Could you check a few things on this model? Use its own coordinates, in mm. A direction names the side the tool comes from. Give positions to 0.01 mm unless a question says otherwise; leave off trailing zeros. Write each loop counter-clockwise with the first axis right and the second up, starting at its lowest first coordinate (ties: lowest second). Pieces come first, ordered by that corner, then holes. Notation, with made-up numbers: (10.5, 69) - (54.5, 69) arc R33 ccw to (54.5, 97) - close; hole circle Ø6 at (-24, -25.75). An arc over 180 degrees is marked (long way). Write item = value, one per line.
from build123d import *

# Parameters (mm, degrees)
F0_W     = 85
F0_H     = 41
F0_R     = 1.8
F0_W_2   = 73
F0_H_2   = 25.4
F1_DEPTH = 3.3
F0_W_3   = 65
F0_H_3   = 15
F2_DEPTH = 5
F3_R     = 5
F4_SIZE  = 3
F5_SIZE  = 1
F6_SIZE  = 1.5


with BuildPart() as f1:
    # F0 (on Top) → F1 (new body)
    with BuildSketch(Plane.XY):
        Rectangle(F0_W, F0_H)
        with Locations((-37.5, -15.5)):
            Circle(F0_R, mode=Mode.SUBTRACT)
        with Locations((37.5, -15.5)):
            Circle(F0_R, mode=Mode.SUBTRACT)
        with Locations((-37.5, 15.5)):
            Circle(F0_R, mode=Mode.SUBTRACT)
        Rectangle(F0_W_2, F0_H_2, mode=Mode.SUBTRACT)
        with Locations((37.5, 15.5)):
            Circle(F0_R, mode=Mode.SUBTRACT)
    extrude(amount=F1_DEPTH)

    # F0 (on Top) → F2 (join)
    with BuildSketch(Plane.XY):
        Rectangle(F0_W, F0_H)
        with Locations((-37.5, -15.5)):
            Circle(F0_R, mode=Mode.SUBTRACT)
        with Locations((37.5, -15.5)):
            Circle(F0_R, mode=Mode.SUBTRACT)
        with Locations((-37.5, 15.5)):
            Circle(F0_R, mode=Mode.SUBTRACT)
        Rectangle(F0_W_2, F0_H_2, mode=Mode.SUBTRACT)
        with Locations((37.5, 15.5)):
            Circle(F0_R, mode=Mode.SUBTRACT)
        Rectangle(F0_W_2, F0_H_2)
        with Locations((0, -1)):
            Rectangle(F0_W_3, F0_H_3, mode=Mode.SUBTRACT)
    extrude(amount=-F2_DEPTH)

    # F3
    f3_edges = [f1.edges().sort_by_distance(p)[0] for p in [
        (-42.5, 20.5, -0.85),
        (-42.5, -20.5, -0.85),
        (42.5, 20.5, -0.85),
        (42.5, -20.5, -0.85),
    ]]
    fillet(f3_edges, radius=F3_R)

    # F4
    f4_edges = [f1.edges().sort_by_distance(p)[0] for p in [
        (0, -8.5, -5),
        (-32.5, -1, -5),
        (0, 6.5, -5),
        (32.5, -1, -5),
    ]]
    chamfer(f4_edges, length=F4_SIZE)

    # F5
    f5_edges = [f1.edges().sort_by_distance(p)[0] for p in [
        (-42.5, 0, -5),
    ]]
    chamfer(f5_edges, length=F5_SIZE)

    # F6
    f6_edges = [f1.edges().sort_by_distance(p)[0] for p in [
        (-39.3, 15.5, -5),
        (-39.3, -15.5, -5),
        (35.7, -15.5, -5),
        (35.7, 15.5, -5),
    ]]
    chamfer(f6_edges, length=F6_SIZE)


solid = f1.part
1. If we section it at C-C, the plane y = 3: Please give me the cut outline in (x, z), and give its area (3 significant figures).
Filled sheet:
outline = (-42.5, -4) - (-41.5, -5) - (-35.5, -5) - (-32.5, -2) - (-32.5, 0) - (-36.5, 0) - (-36.5, 3.3) - (-42.5, 3.3) - close; (32.5, -2) - (35.5, -5) - (41.5, -5) - (42.5, -4) - (42.5, 3.3) - (36.5, 3.3) - (36.5, 0) - (32.5, 0) - close
area = 130 mm2
2. If we section it at A-A, the plane z = 1: Please give me the cut outline in (x, y), and give its area (3 significant figures).
Filled sheet:
outline = (-42.5, -15.5) arc R5 ccw to (-37.5, -20.5) - (37.5, -20.5) arc R5 ccw to (42.5, -15.5) - (42.5, 15.5) arc R5 ccw to (37.5, 20.5) - (-37.5, 20.5) arc R5 ccw to (-42.5, 15.5) - close; hole circle Ø3.6 at (-37.5, -15.5); hole circle Ø3.6 at (-37.5, 15.5); hole (-36.5, -12.7) - (36.5, -12.7) - (36.5, 12.7) - (-36.5, 12.7) - close; hole circle Ø3.6 at (37.5, -15.5); hole circle Ø3.6 at (37.5, 15.5)
area = 1,570 mm2
3. Thinking about a two-plate mould opening in Y: for faces 1 (the face through (-1, -20.5, 0)), 2 (the face through (41.07, 19, -0.4)), 3 (the face through (-1, -13, 3.3)), 4 (the face through (0, 6.5, -1)), which applies, pulls with the +Y half, pulls with the -Y half, needs draft (parallel to the pull), parting line crosses it, or undercut?
Filled sheet:
face_1 = pulls with the -Y half
face_2 = pulls with the +Y half
face_3 = needs draft
face_4 = undercut
4. If we section it at B-B, the plane x = -14: Please give me the cut outline in (y, z), and give its area (3 significant figures).
Filled sheet:
outline = (-20.5, -4) - (-19.5, -5) - (-11.5, -5) - (-8.5, -2) - (-8.5, 0) - (-12.7, 0) - (-12.7, 3.3) - (-20.5, 3.3) - close; (6.5, -2) - (9.5, -5) - (19.5, -5) - (20.5, -4) - (20.5, 3.3) - (12.7, 3.3) - (12.7, 0) - (6.5, 0) - close
area = 171 mm2
5. I need wall thicknesses on line 1 (Y direction, x = 37.5, z = -2.65); line 2 (X direction, y = -3.5, z = -1.25); line 3 (Y direction, x = -14, z = 1.5). Which ranges of each line are inside material? Lowest first, please.
Filled sheet:
line_1 = -20.5 to -17.3, -13.7 to 13.7, 17.3 to 20.5
line_2 = -42.5 to -32.5, 32.5 to 42.5
line_3 = -20.5 to -12.7, 12.7 to 20.5
6. Which directions (+Z, -Z, +X, -X, +Y, -Y) give clear straight access to the entire face, cutting with the end or side of a thin tool? Please do faces 5 (the face through (0, -8.5, -1)), 6 (the face through (42.5, 0, 0)), 7 (the face through (-36.5, 0, 2)), 8 (the face through (-0.5, -10, -3.5)), 9 (the face through (41.07, -19, -0.3)).
Filled sheet:
face_5 = +Z, -Z
face_6 = +Z, -Z, +X, +Y, -Y
face_7 = +Z
face_8 = -Z
face_9 = +Z, -Z, +X, -Y
7. For pin 1 (4.5 mm diameter, centred on x = 37.5, y = -15.5, fed in from +Z); pin 2 (6 mm diameter, centred on x = -37.5, y = -15.5, fed in from -Z); pin 3 (5 mm diameter, centred on x = -31.5, y = 7.5, fed in from +Z), each with a flat end and sliding along its axis, tell me the tip position at first contact or that it passes through.
Filled sheet:
pin_1 = 3.3
pin_2 = -4.7
pin_3 = 0
